from build123d import *

# Parameters (mm, degrees)
F1_DEPTH   = 6.985
F2_R       = 4.1774350827
F3_DEPTH   = 1.27
F6_DEPTH   = 0.508
F8_DEPTH   = 0.508
F9_R       = 1.27
F10_W      = 16.0917048343
F10_H      = 2.0555099472
F8_FACE1_W = 13.7275979897
F8_FACE1_H = 7.493
F11_DEPTH  = 5.08
F12_W      = 10.965348687
F12_H      = 1.5682033263
F13_DEPTH  = 5.08


# Not quite as in the source:
# - a feature names something its author has since deleted; it is built from what else it names


with BuildPart() as f1:
    # F0 (on Front) → F1 (new body)
    with BuildSketch(Plane.XZ):
        Polygon((10.795, 12.6229311572), (-10.795, 12.6229311572), (-8.001, -12.6229311572), (8.001, -12.6229311572), align=None)
    extrude(amount=-F1_DEPTH)

    # F2 (on face) → F3 (join)
    with BuildSketch(Plane.XZ):
        Circle(F2_R)
    extrude(amount=F3_DEPTH)

    # F5 (on face) + F1_face1 (on face) → F6 (join)
    with BuildSketch(Plane.XZ):
        Polygon((-8.0337325091, 0), (-8.597294162, 0), (-7.3735090208, -11.5506481379), (-6.855092685, -11.5506481379), align=None)
    with BuildSketch(Plane(origin=(0, 6.985, 0.6254605528), x_dir=(1, 0, 0), z_dir=(0, 1, 0))):
        Polygon((-10.795, -11.9974706044), (10.795, -11.9974706044), (8.001, 13.2483917101), (-8.001, 13.2483917101), align=None)
    extrude(amount=F6_DEPTH, dir=(0, -1, 0))

    # F7 (on face) → F8 (join)
    with BuildSketch(Plane(origin=(0, 6.985, 0), x_dir=(-1, 0, 0), z_dir=(0, 1, 0))):
        Polygon((8.001, -12.6229311572), (10.795, 12.6229311572), (-10.795, 12.6229311572), (-8.001, -12.6229311572), align=None)
        Polygon((8.051493348, 0), (8.559493348, 0), (7.418411777, -11.551577974), (6.910411777, -11.551577974), align=None, mode=Mode.SUBTRACT)
    extrude(amount=F8_DEPTH)

    # F9
    f9_edges = [f1.edges().sort_by_distance(p)[0] for p in [
        (-10.795, 3.7465, 12.622931),
        (10.795, 3.7465, 12.622931),
        (8.001, 3.7465, -12.622931),
        (-8.001, 3.7465, -12.622931),
    ]]
    fillet(f9_edges, radius=F9_R)

    # F10 (on face) + F8_face1 (on face) → F11 (cut)
    with BuildSketch(Plane.XY.offset(12.6229311572)):
        with Locations((-0.0573594589, 4.0197446942)):
            Rectangle(F10_W, F10_H)
    with BuildSketch(Plane(origin=(0, 3.7465, -12.6229311572), x_dir=(1, 0, 0), z_dir=(0, 0, -1))):
        Rectangle(F8_FACE1_W, F8_FACE1_H)
    extrude(amount=-F11_DEPTH, dir=(0, 0, 1), mode=Mode.SUBTRACT)

    # F12 (on face) → F13 (cut)
    with BuildSketch(Plane(origin=(0, 0, -12.6229311572), x_dir=(1, 0, 0), z_dir=(0, 0, -1))):
        with Locations((-0.0077148434, -3.7751414347)):
            Rectangle(F12_W, F12_H)
    extrude(amount=-F13_DEPTH, mode=Mode.SUBTRACT)


solid = f1.part
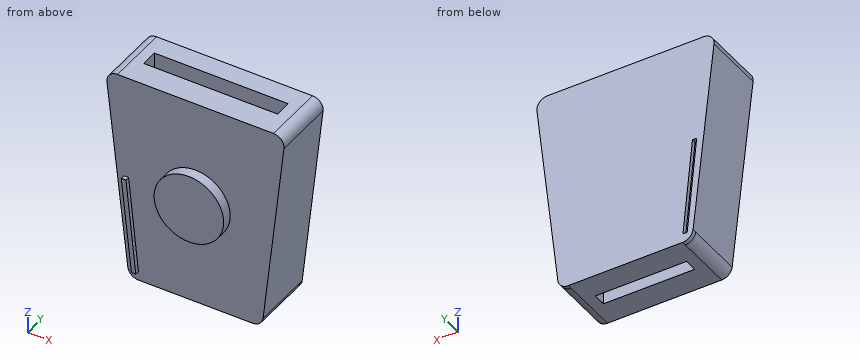
Read the model definition and answer for the solid it produces. Units are mm, in the model's axes. Round coordinates to 2 decimals unless told otherwise and drop trailing zeros. Loops run counter-clockwise (first coordinate to the right, second up) from the corner with the lowest first, then second, coordinate; pieces in that order, holes last. Notation, with made-up numbers: (-12.5, 10) - (7.5, 10) arc R6 cw to (7.5, 19) - close; hole circle Ø10 at (-12, 64). An arc over 180 degrees is marked (long way). One line per question, with ' | ' between items. Start each with the question number.
Q1. Section D-D on y = 1.75 is taken. Give the vertices of the cut face in (x, z).
Q2. Section B-B on x = 0 is taken. Give the vertices of the cut face in (y, z).
Q3. Find the intervals of material crossed by L1, parallel to Y at x = 2.75, z = -10.25; L2, parallel to Y at x = -8, z = 8.75; L3, parallel to Y at x = -3.75, z = 5.5, in increasing order.
Q4. Section A-A on y = 3.5 is taken. Give the vertices of the cut face in (x, z).
Q5. Flat-ended cylindrical pins translate along their axes: pin 1 (1.7 mm diameter, centred on y = 4, z = -9, fed in from +X); pin 2 (1.5 mm diameter, centred on x = -2, z = -7, fed in from -Y); pin 3 (2 mm diameter, centred on y = 2.5, z = 1.5, fed in from -X). Find the tip coordinate at first contact, or state that the pin passes through.
Q6. Section C-C on z = -6.75 is taken. Give the vertices of the cut face in (x, y) (3 decimals), plus the area to 3 significant figures.
Established:
1) outline: (-10.64, 11.21) - (-8.13, -11.49) arc R1.27 ccw to (-6.86, -12.62) - (6.86, -12.62) arc R1.27 ccw to (8.13, -11.49) - (10.64, 11.21) arc R1.27 ccw to (9.38, 12.62) - (-9.38, 12.62) arc R1.27 ccw to start
2) outline: (-1.27, -4.18) - (0, -4.18) - (0, -12.62) - (2.99, -12.62) - (2.99, -7.54) - (4.56, -7.54) - (4.56, -12.62) - (7.49, -12.62) - (7.49, 12.62) - (5.05, 12.62) - (5.05, 7.54) - (2.99, 7.54) - (2.99, 12.62) - (0, 12.62) - (0, 4.18) - (-1.27, 4.18) - close
3) L1: 0 to 2.99, 4.56 to 7.49 | L2: 0 to 2.99, 5.05 to 7.49 | L3: 0 to 7.49
4) outline: (-10.64, 11.21) - (-8.13, -11.49) arc R1.27 ccw to (-6.86, -12.62) - (-5.49, -12.62) - (-5.49, -7.54) - (5.47, -7.54) - (5.47, -12.62) - (6.86, -12.62) arc R1.27 ccw to (8.13, -11.49) - (10.64, 11.21) arc R1.27 ccw to (9.38, 12.62) - (7.99, 12.62) - (7.99, 7.54) - (-8.1, 7.54) - (-8.1, 12.62) - (-9.38, 12.62) arc R1.27 ccw to start
5) pin 1: x = 8.5 | pin 2: y = 0 | pin 3: x = -9.67
6) outline: (-8.651, 0) - (-7.882, 0) - (-7.882, -0.508) - (-7.345, -0.508) - (-7.345, 0) - (8.651, 0) - (8.651, 7.493) - (-7.385, 7.493) - (-7.385, 6.985) - (-7.893, 6.985) - (-7.893, 7.493) - (-8.651, 7.493) - close | area: 130 mm²
